```python
from build123d import *

# Parameters (mm, degrees)
F1_DEPTH = 101.6
F2_DEPTH = 25.4
F3_W     = 25.4
F3_H     = 50.747624588
F4_DEPTH = 38.1


with BuildPart() as f1:
    # F0 (on Front) → F1 (new body)
    with BuildSketch(Plane.XZ):
        Polygon((-40.3379746149, -16.229630179), (-40.3379746149, -41.629630179), (23.1620253851, -41.629630179), (23.1620253851, 34.570369821), (-14.9379746149, 34.570369821), (-14.9379746149, -16.229630179), align=None)
    extrude(amount=F1_DEPTH)

    # F2 (add): a face of the model
    f2_faces = [f1.faces().sort_by_distance(p)[0] for p in [
        (4.1120253851, -50.8, 34.570369821),
    ]]
    extrude(f2_faces, amount=F2_DEPTH)

    # F3 (on face) → F4 (cut)
    with BuildSketch(Plane.XY.offset(59.970369821)):
        with Locations((-2.2379746149, -50.826187706)):
            Rectangle(F3_W, F3_H)
    extrude(amount=-F4_DEPTH, mode=Mode.SUBTRACT)


solid = f1.part
```
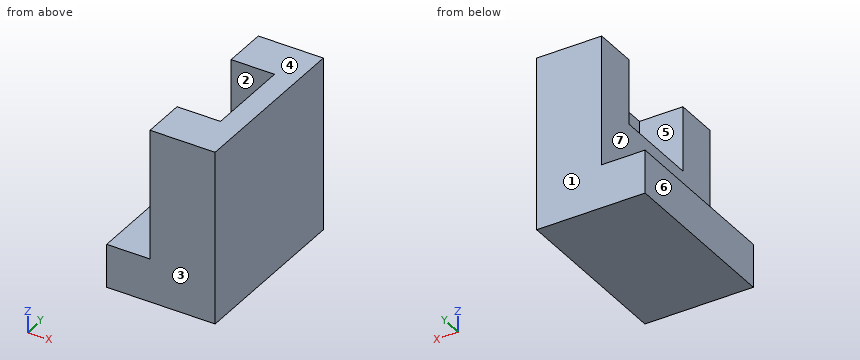
Input: part model. Units: mm. Frame: model coordinates. Face numbers are marked on the shaded views. A direction names the side the tool comes from. Coordinates: 2 decimals unless noted, no trailing zeros. Write each loop counter-clockwise with the first axis right and the second up, starting at its lowest first coordinate (ties: lowest second). Pieces come first, ordered by that corner, then holes. Notation, with made-up numbers: (59.25, -13.5) - (117.25, -13.5) arc R25 cw to (117.25, 18.5) - close; hole circle Ø7 at (65.25, -30). An arc over 180 degrees is marked (long way). Put each result on its own line as item: value. Start each with the question number.
1) Reachability of the marked faces 5, 6 and 7 from +Z, -Z, +X, -X, +Y, -Y: full face, straight path, thin tool, end or side. Return the list, or none.
2) Cut plane A-A (y = -65). Return the cut outline in (x, z), plus the area to 3 significant figures.
3) Cut plane D-D (x = -33). Return the cut outline in (y, z).
4) Ray query, L1, parallel to X at y = -63.5, z = 53.5; L2, parallel to Y at x = 6.5, z = 28; L3, parallel to X at y = -90.5, z = -11.5. Return the intervals inside material, ascending.
5) Contact query for flat-ended pins moving along their axis: pin 1 (5 mm diameter, centred on x = -12.5, y = -47, fed in from +Z); pin 2 (19 mm diameter, centred on y = -40, z = 38.5, fed in from -X); pin 3 (3 mm diameter, centred on y = -45.5, z = -11.5, fed in from -X). Output: stop coordinate, or through.
6) Cut plane C-C (z = 6.5). Return the cut outline in (x, y), plus the area to 3 significant figures.
7) Mould query, pull axis Y, two halves, no side actions, for the marked faces 1, 2, 3 and 4. Classes: pulls with the +Y half, pulls with the -Y half, needs draft (parallel to the pull), parting line crosses it, or undercut.
8) Cut plane B-B (x = -5). Return the cut outline in (y, z).
Resolved:
1. face 5: +Z, -X
1. face 6: +Z, -Z, -X, +Y, -Y
1. face 7: +Z, -X, +Y, -Y
2. outline: (-40.34, -41.63) - (23.16, -41.63) - (23.16, 59.97) - (10.46, 59.97) - (10.46, 21.87) - (-14.94, 21.87) - (-14.94, -16.23) - (-40.34, -16.23) - close
2. area: 3,550 mm2
3. outline: (-101.6, -41.63) - (0, -41.63) - (0, -16.23) - (-101.6, -16.23) - close
4. L1: x = 10.46 to 23.16
4. L2: y = -101.6 to -76.2, -25.45 to 0
4. L3: x = -14.94 to 23.16
5. pin 1: stops at z = 21.87
5. pin 2: stops at x = 10.46
5. pin 3: stops at x = -14.94
6. outline: (-14.94, -101.6) - (23.16, -101.6) - (23.16, 0) - (-14.94, 0) - close
6. area: 3,870 mm2
7. face 1: pulls with the +Y half
7. face 2: undercut
7. face 3: pulls with the -Y half
7. face 4: needs draft
8. outline: (-101.6, -41.63) - (0, -41.63) - (0, 59.97) - (-25.45, 59.97) - (-25.45, 21.87) - (-76.2, 21.87) - (-76.2, 59.97) - (-101.6, 59.97) - close
